Verification items for this drawing (mm, ordinates from the low corner). A direction names the side the tool comes from. Round coordinates to 2 decimals unless told otherwise and drop trailing zeros. Order: outer loops, then holes, each group sorted by start corner. A loop starts at its lowest first (then second) coordinate and runs counter-clockwise, first axis right, second up. Notation, with made-up numbers: (-19, 24) -> (10, 24) arc R11 ccw to (10, 42) -> close; hole circle Ø11 at (-13.75, 82.5). An arc over 180 degrees is marked (long way). Answer in a Markdown table with one row per item.
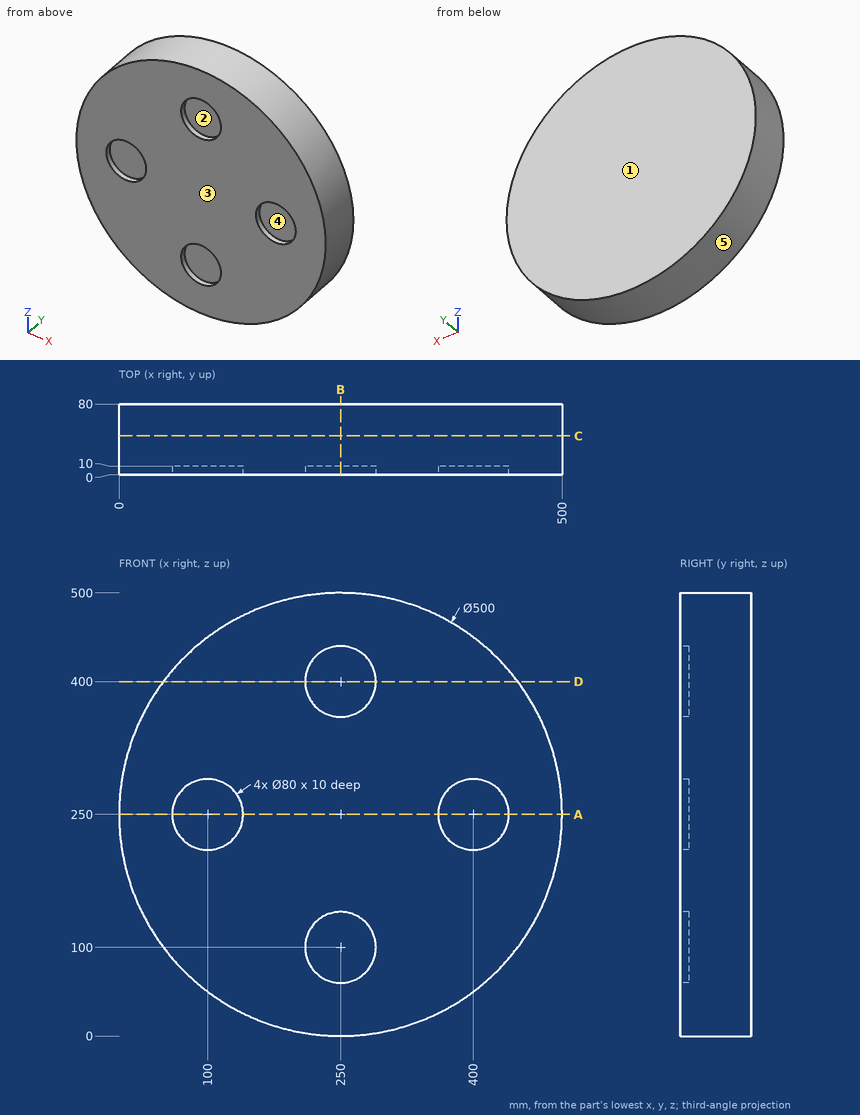
Item 1: Cross-section at D-D (z = 400). Record the boundary of the cut face in (x, y), and give its area (3 significant figures).
Result sheet:
| item | result |
|---|---|
| outline | (50, 0) -> (210, 0) -> (210, 10) -> (290, 10) -> (290, 0) -> (450, 0) -> (450, 80) -> (50, 80) -> close |
| area | 31,200 mm^2 |
Item 2: Set-up check for the marked faces 1 and 2: record each of +Z, -Z, +X, -X, +Y, -Y from which the full face is reachable in a straight line by a thin tool's end or side.
Result sheet:
| item | result |
|---|---|
| face 1 | +Z, -Z, +X, -X, +Y |
| face 2 | -Y |
Item 3: Cross-section at B-B (x = 250). Record the boundary of the cut face in (y, z).
Result sheet:
| item | result |
|---|---|
| outline | (0, 0) -> (80, 0) -> (80, 500) -> (0, 500) -> (0, 440) -> (10, 440) -> (10, 360) -> (0, 360) -> (0, 140) -> (10, 140) -> (10, 60) -> (0, 60) -> close |
Item 4: Depth check by flat-ended pin: P1, Ø10, axis at x = 126, y = 50, coming from the -Z side; P2, Ø1.5, axis at x = 327.5, y = 23.5, coming from the +Z side; P3, Ø24, axis at x = 104.5, z = 261, coming from the -Y side. Enter the tip coordinate at first touch or a pass-through.
Result sheet:
| item | result |
|---|---|
| P1 | stops at z = 30.14 |
| P2 | stops at z = 487.93 |
| P3 | stops at y = 10 |
Item 5: Cross-section at C-C (y = 44). Record the boundary of the cut face in (x, z).
Result sheet:
| item | result |
|---|---|
| outline | circle Ø500 at (250, 250) |
Item 6: Scan lines: line 1 (Z direction, x = 250, y = 2); line 2 (Z direction, x = 100, y = 6.75); line 3 (X direction, y = 8, z = 423). Record each from-to range of solid material in increasing order. Write a range as [from, to].
Result sheet:
| item | result |
|---|---|
| line 1 | z = [0, 60], [140, 360], [440, 500] |
| line 2 | z = [50, 210], [290, 450] |
| line 3 | x = [69.53, 217.27], [282.73, 430.47] |
Item 7: Cross-section at A-A (z = 250). Record the boundary of the cut face in (x, y), and give its area (3 significant figures).
Result sheet:
| item | result |
|---|---|
| outline | (0, 0) -> (60, 0) -> (60, 10) -> (140, 10) -> (140, 0) -> (360, 0) -> (360, 10) -> (440, 10) -> (440, 0) -> (500, 0) -> (500, 80) -> (0, 80) -> close |
| area | 38,400 mm^2 |
Item 8: Mould release check, pull along X, two halves, no side actions. Record for the marked faces 3, 4 and 5: pulls with the +X half, pulls with the -X half, needs draft (parallel to the pull), parting line crosses it, or undercut.
Result sheet:
| item | result |
|---|---|
| face 3 | needs draft |
| face 4 | undercut |
| face 5 | parting line crosses it |
